from build123d import *

# Parameters (mm, degrees)
BOSS_EXTRUDE1_DEPTH = 22.5
CUT_EXTRUDE1_DEPTH  = 128.008857959


with BuildPart() as part:
    # Sketch1 → Boss-Extrude1 (new, symmetric)
    with BuildSketch(Plane.XY):
        with BuildLine():
            Line((-17.5, 118.717100706), (-17.5, 30.31))
            Line((-17.5, 30.31), (17.5, 30.31))
            Line((17.5, 30.31), (17.5, 118.717100706))
            ThreePointArc((17.5, 118.717100706), (0, 120), (-17.5, 118.717100706))
        make_face()
    extrude(amount=BOSS_EXTRUDE1_DEPTH, both=True)

    # Sketch2 → Cut-Extrude1 (cut, through all)
    with BuildSketch(Plane(origin=(17.5, 0, 0), x_dir=(0, 0, -1), z_dir=(1, 0, 0))):
        Polygon((-22.5, 54.019237886), (-7.5, 80), (-7.5, 120), (-22.5, 120), align=None)
    extrude(amount=-CUT_EXTRUDE1_DEPTH, mode=Mode.SUBTRACT)


solid = part.part
Verification items for the finished model (mm, model axes). A direction names the side the tool comes from. Give positions to 0.01 mm unless a question says otherwise; leave off trailing zeros. Loops run counter-clockwise (first coordinate to the right, second up) from the corner with the lowest first, then second, coordinate; pieces in that order, holes last.
1. Cross-section at D-D on x = -5. Record the cut outline in (y, z).
Derived:
outline: (30.31, -22.5) - (119.9, -22.5) - (119.9, 7.5) - (80, 7.5) - (54.02, 22.5) - (30.31, 22.5) - close
2. Go/stop test with flat-tipped pins: P1, Ø6, axis at x = -10.5, z = -15, coming from the +Y side; P2, Ø1.5, axis at x = -6.5, z = -13.5, coming from the +Y side; P3, Ø5, axis at x = -6.5, z = 17, coming from the +Y side. Record where each tip stops, or that it passes through.
Derived:
P1: stops at y = 119.77
P2: stops at y = 119.86
P3: stops at y = 67.88
3. Material ranges on probe 1 along Y at (x, z) = (0, -10.5); probe 2 along Z at (x, y) = (11, 80.5); probe 3 along Y at (x, z) = (-12.5, 3), recorded low to high.
Derived:
probe 1: y = 30.31 to 120
probe 2: z = -22.5 to 7.5
probe 3: y = 30.31 to 119.35
4. Cross-section at C-C on z = 18. Record the cut outline in (x, y), and give its area (3 significant figures).
Derived:
outline: (-17.5, 30.31) - (17.5, 30.31) - (17.5, 61.81) - (-17.5, 61.81) - close
area: 1,100 mm2
5. Tool access check on faces 1 (the flat face through (0, 30.31, 0)), 2 (the flat face through (0, 100, 7.5)). Record the directions out of +Z, -Z, +X, -X, +Y, -Y that give a thin tool (end or side, any length) a straight path to the whole face; none if there is none.
Derived:
face 1: +Z, -Z, +X, -X, -Y
face 2: +Z, +X, -X, +Y
6. Cross-section at A-A on x = 2.5. Record the cut outline in (y, z), and give its area (3 significant figures).
Derived:
outline: (30.31, -22.5) - (119.97, -22.5) - (119.97, 7.5) - (80, 7.5) - (54.02, 22.5) - (30.31, 22.5) - close
area: 3,240 mm2
7. Cross-section at B-B on y = 87. Record the cut outline in (x, z), and give its area (3 significant figures).
Derived:
outline: (-17.5, -22.5) - (17.5, -22.5) - (17.5, 7.5) - (-17.5, 7.5) - close
area: 1,050 mm2
